Can you work these out from the model? Positions are in its coordinate system, mm. Coordinates: 2 decimals unless noted, no trailing zeros. Order: outer loops, then holes, each group sorted by start corner. A loop starts at its lowest first (then second) coordinate and runs counter-clockwise, first axis right, second up. Notation, with made-up numbers: (6.5, 8.5) -> (21.5, 8.5) arc R12 cw to (21.5, 22.5) -> close; hole circle Ø10 at (17.5, 26.25). An arc over 180 degrees is marked (long way). Write item = value, one per line.
```python
from build123d import *

# Parameters (mm, degrees)
ESBO_O1_W                = 25
ESBO_O1_H                = 25
RESSALTO_EXTRUS_O3_DEPTH = 3


with BuildPart() as part:
    # Esboço1 → Ressalto-extrusão3 (new body)
    with BuildSketch(Plane(origin=(0, 0, 0), x_dir=(1, 0, 0), z_dir=(0, 1, 0))):
        Polygon((0, 91), (0, 0), (25, 0), (25, 3), (55, 3), (55, 0), (179, 0), (179, 3), (209, 3), (209, 0), (234, 0), (234, 91), (231, 91), (231, 141), (234, 141), (234, 232), (209, 232), (209, 229), (179, 229), (179, 232), (55, 232), (55, 229), (25, 229), (25, 232), (0, 232), (0, 141), (3, 141), (3, 91), align=None)
        with Locations((115.5, 105)):
            Rectangle(ESBO_O1_W, ESBO_O1_H, mode=Mode.SUBTRACT)
    extrude(amount=RESSALTO_EXTRUS_O3_DEPTH)


solid = part.part
```
Item 1: I'm going to push flat-ended pins straight in: P1, Ø1.5, axis at y = 2, z = -116.5, coming from the -X side; P2, Ø1.5, axis at x = 33.5, y = 2, coming from the -Z side. Where does each tip first touch, or does it pass through?
A:
P1 = 3
P2 = -229
Item 2: I want a section at C-C, the plane x = 196. Please give me the cut outline in (y, z), plus the area to 3 significant figures.
A:
outline = (0, -229) -> (3, -229) -> (3, -3) -> (0, -3) -> close
area = 678 mm2
Item 3: I want a section at B-B, the plane z = -125. Please give me the cut outline in (x, y), plus the area to 3 significant figures.
A:
outline = (3, 0) -> (231, 0) -> (231, 3) -> (3, 3) -> close
area = 684 mm2
Item 4: If I drill on probe 1 along X at (y, z) = (0.7, -114); probe 2 along Z at (x, y) = (186.5, 1.8); probe 3 along Z at (x, y) = (121.5, 2), over which ranges is the centre line in solid material (lowest first)?
A:
probe_1 = 3 to 103, 128 to 231
probe_2 = -229 to -3
probe_3 = -232 to -117.5, -92.5 to 0
